The listing builds one solid part. Answer for the finished solid, in the listing's coordinates (mm). A direction names the side the tool comes from. Give positions to 0.01 mm unless a question says otherwise; leave off trailing zeros. Write each loop counter-clockwise with the first axis right and the second up, starting at its lowest first coordinate (ties: lowest second). Pieces come first, ordered by that corner, then holes. Notation, with made-up numbers: (-18, 55.25) - (3, 55.25) arc R19 cw to (3, 64.25) - close; hole circle Ø5 at (-17.75, 19.5). An arc over 180 degrees is marked (long way). One line per question, with ' | ' between items. Start each with the question number.
1. Given P1, Ø3.5, axis at x = 12, z = 0, coming from the +Y side, flat-ended and moving along its own axis, determine where the tip first touches the part or whether it passes through.
2. Find the intervals of material crossed by L1, parallel to Z at x = 132, y = -0.35; L2, parallel to Z at x = 42, y = 1.65; L3, parallel to Y at x = 117.5, z = -1.75, in increasing order. Write a range as from..to.
3. A cutting plane is placed at A-A (x = 87). Determine the outline of the cut face in (y, z), then the cut area to 3 significant figures.
4. A cutting plane is placed at C-C (x = 18.5). Determine the outline of the cut face in (y, z).
5. The mould has two halves that part along X. Classify faces 1 (the face through (58.11, -1.13, 0.46)), 2 (the face through (71, -2.396, 1)), 3 (the face through (144, 0, 0)): +X half, -X half, draft (parallel to the pull), parting line (faces both ways), or undercut.
6. A cutting plane is placed at B-B (y = -0.9). State how many separate pieces and enclosed holes the cut face has, then the cut area to 3 significant figures.
7. For faces 4 (the face through (28, 0.1, 1)), 5 (the face through (88.11, -1.13, 0.46)), determine the directions among +Z, -Z, +X, -X, +Y, -Y from which every point of the face is accessible in a straight line to the end or side of a thin tool.
```python
from build123d import *

# Parameters (mm, degrees)
EXTRUDE_1_DEPTH          = 144
SKETCH_2_R               = 2.1
CUT_EXTRUDE_1_DEPTH      = 2.3
SKETCH_3_R               = 1.2
CUT_EXTRUDE_2_DEPTH      = 1
CUT_EXTRUDE_2_DEPTH_BACK = 5.795979797


with BuildPart() as part:
    # 草图1 → 凸台-拉伸1 (new body)
    with BuildSketch(Plane(origin=(0, 0, 0), x_dir=(0, 0, -1), z_dir=(1, 0, 0))):
        with BuildLine():
            Line((3.497989899, 0.202010101), (3.497989899, -2.197989899))
            Line((3.497989899, -2.197989899), (3.3, -2.395979797))
            Line((3.3, -2.395979797), (-3.3, -2.395979797))
            Line((-3.3, -2.395979797), (-3.497989899, -2.197989899))
            Line((-3.497989899, -2.197989899), (-3.497989899, 0.202010101))
            ThreePointArc((-3.497989899, 0.202010101), (-2.797989899, 0.902010101), (-3.497989899, 1.602010101))
            Line((-3.497989899, 1.602010101), (-3.497989899, 2.202010101))
            Line((-3.497989899, 2.202010101), (-3.3, 2.4))
            Line((-3.3, 2.4), (3.3, 2.4))
            Line((3.3, 2.4), (3.497989899, 2.202010101))
            Line((3.497989899, 2.202010101), (3.497989899, 1.602010101))
            ThreePointArc((3.497989899, 1.602010101), (2.797989899, 0.902010101), (3.497989899, 0.202010101))
        make_face()
    extrude(amount=EXTRUDE_1_DEPTH)

    # 草图2 → 切除-拉伸1 (cut)
    with BuildSketch(Plane(origin=(0, 2.4, 0), x_dir=(1, 0, 0), z_dir=(0, 1, 0))):
        with Locations((12, 0)):
            Circle(SKETCH_2_R)
        with Locations((27, 0)):
            Circle(SKETCH_2_R)
        with Locations((42, 0)):
            Circle(SKETCH_2_R)
        with Locations((57, 0)):
            Circle(SKETCH_2_R)
        with Locations((72, 0)):
            Circle(SKETCH_2_R)
        with Locations((87, 0)):
            Circle(SKETCH_2_R)
        with Locations((102, 0)):
            Circle(SKETCH_2_R)
        with Locations((117, 0)):
            Circle(SKETCH_2_R)
        with Locations((132, 0)):
            Circle(SKETCH_2_R)
        with Locations((147, 0)):
            Circle(SKETCH_2_R)
        with Locations((162, 0)):
            Circle(SKETCH_2_R)
        with Locations((177, 0)):
            Circle(SKETCH_2_R)
        with Locations((192, 0)):
            Circle(SKETCH_2_R)
        with Locations((207, 0)):
            Circle(SKETCH_2_R)
        with Locations((222, 0)):
            Circle(SKETCH_2_R)
    extrude(amount=-CUT_EXTRUDE_1_DEPTH, mode=Mode.SUBTRACT)

    # 草图3 → 切除-拉伸2 (cut, two sides)
    with BuildSketch(Plane(origin=(0, 2.4, 0), x_dir=(1, 0, 0), z_dir=(0, 1, 0))) as cut_extrude_2_sk:
        with Locations((12, 0)):
            Circle(SKETCH_3_R)
        with Locations((27, 0)):
            Circle(SKETCH_3_R)
        with Locations((42, 0)):
            Circle(SKETCH_3_R)
        with Locations((57, 0)):
            Circle(SKETCH_3_R)
        with Locations((72, 0)):
            Circle(SKETCH_3_R)
        with Locations((87, 0)):
            Circle(SKETCH_3_R)
        with Locations((102, 0)):
            Circle(SKETCH_3_R)
        with Locations((117, 0)):
            Circle(SKETCH_3_R)
        with Locations((132, 0)):
            Circle(SKETCH_3_R)
        with Locations((147, 0)):
            Circle(SKETCH_3_R)
        with Locations((162, 0)):
            Circle(SKETCH_3_R)
        with Locations((177, 0)):
            Circle(SKETCH_3_R)
        with Locations((192, 0)):
            Circle(SKETCH_3_R)
        with Locations((207, 0)):
            Circle(SKETCH_3_R)
        with Locations((222, 0)):
            Circle(SKETCH_3_R)
    extrude(amount=CUT_EXTRUDE_2_DEPTH, mode=Mode.SUBTRACT)
    extrude(cut_extrude_2_sk.sketch, amount=-CUT_EXTRUDE_2_DEPTH_BACK, mode=Mode.SUBTRACT)


solid = part.part
```
Determined:
1) P1: y = 0.1
2) L1: -3.5..-1.2, 1.2..3.5 | L2: -3.5..-2.1, 2.1..3.5 | L3: -2.4..0.1
3) outline: (-2.4, -3.3) - (-2.2, -3.5) - (0.2, -3.5) arc R0.7 cw to (1.6, -3.5) - (2.2, -3.5) - (2.4, -3.3) - (2.4, -2.1) - (0.1, -2.1) - (0.1, -1.2) - (-2.4, -1.2) - close; (-2.4, 1.2) - (0.1, 1.2) - (0.1, 2.1) - (2.4, 2.1) - (2.4, 3.3) - (2.2, 3.5) - (1.6, 3.5) arc R0.7 cw to (0.2, 3.5) - (-2.2, 3.5) - (-2.4, 3.3) - close | area: 16.3 mm2
4) outline: (-2.4, -3.3) - (-2.2, -3.5) - (0.2, -3.5) arc R0.7 cw to (1.6, -3.5) - (2.2, -3.5) - (2.4, -3.3) - (2.4, 3.3) - (2.2, 3.5) - (1.6, 3.5) arc R0.7 cw to (0.2, 3.5) - (-2.2, 3.5) - (-2.4, 3.3) - close
5) face 1: undercut | face 2: draft | face 3: +X half
6) separate pieces: 1 | enclosed holes: 9 | area: 967 mm2
7) face 4: +Y | face 5: +Y, -Y
